from build123d import *

# Parameters (mm, degrees)
SKETCH1_R           = 40
BOSS_EXTRUDE1_DEPTH = 14
SKETCH2_R           = 1.5
CUT_EXTRUDE1_DEPTH  = 76.584389923
CIRPATTERN1_COUNT   = 8
SKETCH5_W           = 108
SKETCH5_H           = 14
BOSS_EXTRUDE2_DEPTH = 8


with BuildPart() as part:
    # Sketch1 → Boss-Extrude1 (new body)
    with BuildSketch(Plane.XY):
        with BuildLine():
            Line((46, -46), (54, -46))
            Line((54, -46), (54, -51))
            Line((54, -51), (-54, -51))
            Line((-54, -51), (-54, -46))
            Line((-54, -46), (-46, -46))
            Line((-46, -46), (-46, 0))
            ThreePointArc((-46, 0), (0, 46), (46, 0))
            Line((46, 0), (46, -46))
        make_face()
        Circle(SKETCH1_R, mode=Mode.SUBTRACT)
    extrude(amount=BOSS_EXTRUDE1_DEPTH)

    # Sketch2 → Cut-Extrude1 (cut, through all)
    with BuildSketch(Plane(origin=(0, 0, 0), x_dir=(1, 0, 0), z_dir=(0, 1, 0))):
        with Locations(Location((0, -7, 0), (0, 0, 90))):
            Circle(SKETCH2_R)
    cut_extrude1 = extrude(amount=CUT_EXTRUDE1_DEPTH, mode=Mode.SUBTRACT)

    # CirPattern1: Cut-Extrude1 ×8 about axis
    cirpattern1_axis = Axis((0, 0, 0), (0, 0, 1))
    for i in range(1, CIRPATTERN1_COUNT):
        add(cut_extrude1.rotate(cirpattern1_axis, i * 360 / CIRPATTERN1_COUNT), mode=Mode.SUBTRACT)

    # Sketch5 → Boss-Extrude2 (add)
    with BuildSketch(Plane.XZ.offset(51)):
        with Locations((0, 7)):
            Rectangle(SKETCH5_W, SKETCH5_H)
    extrude(amount=-BOSS_EXTRUDE2_DEPTH)


solid = part.part
Read the model definition and answer for the solid it produces. Units are mm, in the model's axes. A direction names the side the tool comes from. Give positions to 0.01 mm unless a question says otherwise; leave off trailing zeros. Write each loop counter-clockwise with the first axis right and the second up, starting at its lowest first coordinate (ties: lowest second). Pieces come first, ordered by that corner, then holes. Notation, with made-up numbers: (49, 65.5) - (84, 65.5) arc R13 ccw to (84, 86.5) - close; hole circle Ø1 at (5, -28). An arc over 180 degrees is marked (long way). Return JSON: item names as keys, results as strings.
Q1. For a pull along Y with two mould halves and no side action, classify faces 6 (the face through (8, -42, 0)), 7 (the face through (42.94, 0.07, 8.5)), 8 (the face through (1, -51, 7)) as released by +Y, released by -Y, zero draft, split by the parting line, or undercut.
Reply:
{"face 6": "zero draft", "face 7": "undercut", "face 8": "released by -Y"}
Q2. A cutting plane is placed at C-C, the plane y = -8. Determine the outline of the cut face in (x, z).
Reply:
{"outline": "(-46, 0) - (-39.19, 0) - (-39.19, 14) - (-46, 14) - close; (39.19, 0) - (46, 0) - (46, 14) - (39.19, 14) - close"}
Q3. For faces 1 (the face through (-0.07, 42.94, 8.5)), 2 (the face through (46, -21, 7)), 3 (the face through (-43, -43, 7)), 4 (the face through (-50, -43, 7)), 5 (the face through (-8.67, -39.05, 6.9)), determine the directions among +Z, -Z, +X, -X, +Y, -Y from which every point of the face is accessible in a straight line to the end or side of a thin tool.
Reply:
{"face 1": "+Y", "face 2": "+Z, -Z, +X, +Y", "face 3": "none", "face 4": "+Z, -Z, -X, +Y", "face 5": "+Z, -Z"}
Q4. Consider line 1 along X through (y, z) = (-41.35, 7); line 2 along X through (y, z) = (-41.4, 7); line 3 along Y through (x, z) = (0, 3.5). Determine where each line is inside the solid, lowest interval first. Write a range as [from, to].
Reply:
{"line 1": "[-46, -43.47], [-39.23, -1.5], [1.5, 39.23], [43.47, 46]", "line 2": "[-46, -43.52], [-39.28, -1.5], [1.5, 39.28], [43.52, 46]", "line 3": "[-51, -40], [40, 46]"}
Q5. A cutting plane is placed at D-D, the plane x = 23.5. Determine the outline of the cut face in (y, z), and give its area (3 significant figures).
Reply:
{"outline": "(-51, 0) - (-32.37, 0) - (-32.37, 14) - (-51, 14) - close; (32.37, 0) - (39.54, 0) - (39.54, 14) - (32.37, 14) - close", "area": "361 mm²"}
Q6. A cutting plane is placed at A-A, the plane x = 0. Determine the outline of the cut face in (y, z).
Reply:
{"outline": "(-51, 0) - (-40, 0) - (-40, 5.5) - (-43, 5.5) - (-43, 8.5) - (-40, 8.5) - (-40, 14) - (-51, 14) - close; (40, 0) - (46, 0) - (46, 5.5) - (40, 5.5) - close; (40, 8.5) - (46, 8.5) - (46, 14) - (40, 14) - close"}
Q7. A cutting plane is placed at B-B, the plane z = 10.5. Determine the outline of the cut face in (x, y), and give its area (3 significant figures).
Reply:
{"outline": "(-54, -51) - (54, -51) - (54, -43) - (46, -43) - (46, 0) arc R46 ccw to (-46, 0) - (-46, -43) - (-54, -43) - close; hole circle Ø80 at (0, 0)", "area": "3,120 mm²"}
Q8. Given P1, Ø2, axis at y = 21.5, z = 7.5, coming from the -X side; P2, Ø2, axis at x = -32, z = 3.5, coming from the +Y side; P3, Ø4, axis at x = -52, z = 5.5, coming from the +Y side; P4, Ø3, axis at x = 35.5, y = 33, coming from the -Z side, each flat-ended and moving along its own axis, determine where each tip first touches the part or whether it passes through.
Reply:
{"P1": "x = -41.18", "P2": "y = 33.99", "P3": "y = -43", "P4": "through"}
